Here's how the part is built. I have some questions about the finished solid (model axes, mm). Face numbers are marked on the shaded views. A direction names the side the tool comes from. Coordinates: 2 decimals unless noted, no trailing zeros. Loops run counter-clockwise (first coordinate to the right, second up) from the corner with the lowest first, then second, coordinate; pieces in that order, holes last. Notation, with made-up numbers: (3, 75) -> (54, 75) arc R23 cw to (54, 91) -> close; hole circle Ø6 at (36, 84). An arc over 180 degrees is marked (long way). Answer as a JSON object with one key per item and string values. Group by question number.
Q1. I want a section at B-B on y = 119.5. Write out the boundary of the cut face in (x, z).
Q2. I'm going to push flat-ended pins straight in: pin 1 (6 mm diameter, centred on x = 66, y = 139.5, fed in from -Z); pin 2 (8 mm diameter, centred on x = -52, y = -66, fed in from +Z). Where does each tip first touch, or does it pass through?
Q3. On a 3-axis mill with a long thin cutter (end or side, diameter ignored), from which of +Z, -Z, +X, -X, +Y, -Y can I reach the whole of each face in a straight line? I mean the marked faces 5 and 6. Say none if no direction works.
Q4. I want a section at A-A on z = 96. Write out the boundary of the cut face in (x, y), then the cut area to 3 significant figures.
Q5. I want a section at C-C on x = -93.5. Write out the boundary of the cut face in (y, z), then the cut area to 3 significant figures.
Q6. I need wall thicknesses on line 1 (X direction, y = 207, z = 84); line 2 (Y direction, x = 89.5, z = 202); line 3 (Y direction, x = -180.5, z = 237.5). Which ranges of each line are inside material? Lowest first, please.
Q7. Thinking about a two-plate mould opening in Y: for the marked faces 1, 2, 3 and 4, which applies, released by +Y, released by -Y, zero draft, split by the parting line, or undercut?
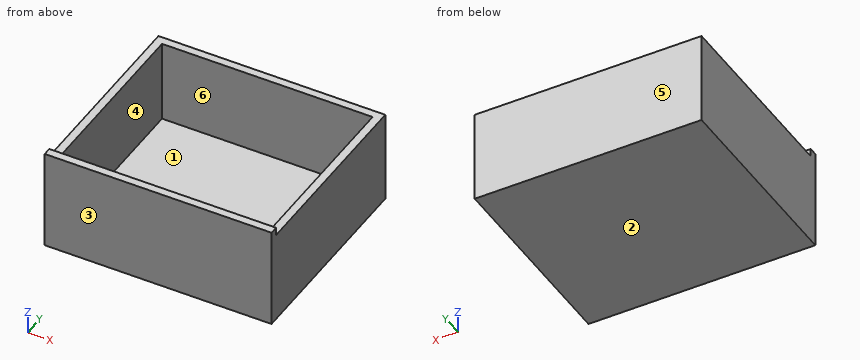
```python
from build123d import *

# Parameters (mm, degrees)
F0_W     = 20
F0_H     = 460
F0_H_2   = 20
F0_W_2   = 520
F1_DEPTH = 230
F2_DEPTH = 250
F3_DEPTH = 25


with BuildPart() as f1:
    # F0 (on Top) → F1 (new body)
    with BuildSketch(Plane.XY):
        with Locations((-270, 0)):
            Rectangle(F0_W, F0_H)
        with Locations((-270, 240)):
            Rectangle(F0_W, F0_H_2)
        with Locations((0, 240)):
            Rectangle(F0_W_2, F0_H_2)
        with Locations((270, 0)):
            Rectangle(F0_W, F0_H)
        with Locations((270, 240)):
            Rectangle(F0_W, F0_H_2)
    extrude(amount=F1_DEPTH)

    # F0 (on Top) → F2 (join)
    with BuildSketch(Plane.XY):
        with Locations((-270, -240)):
            Rectangle(F0_W, F0_H_2)
        with Locations((0, -240)):
            Rectangle(F0_W_2, F0_H_2)
        with Locations((270, -240)):
            Rectangle(F0_W, F0_H_2)
    extrude(amount=F2_DEPTH)

    # F0 (on Top) → F3 (join)
    with BuildSketch(Plane.XY):
        with Locations((270, -240)):
            Rectangle(F0_W, F0_H_2)
        with Locations((0, -240)):
            Rectangle(F0_W_2, F0_H_2)
        with Locations((270, 0)):
            Rectangle(F0_W, F0_H)
        with Locations((-270, -240)):
            Rectangle(F0_W, F0_H_2)
        with Locations((270, 240)):
            Rectangle(F0_W, F0_H_2)
        with Locations((-270, 0)):
            Rectangle(F0_W, F0_H)
        with Locations((0, 240)):
            Rectangle(F0_W_2, F0_H_2)
        with Locations((-270, 240)):
            Rectangle(F0_W, F0_H_2)
        Rectangle(F0_W_2, F0_H)
    extrude(amount=F3_DEPTH)


solid = f1.part
```
Result set:
{
 "1": {"outline": "(-280, 0) -> (280, 0) -> (280, 230) -> (260, 230) -> (260, 25) -> (-260, 25) -> (-260, 230) -> (-280, 230) -> close"},
 "2": {"pin 1": "stops at z = 0", "pin 2": "stops at z = 25"},
 "3": {"face 5": "+Z, -Z, +X, -X, +Y", "face 6": "+Z"},
 "4": {"outline": "(-280, -250) -> (280, -250) -> (280, 250) -> (-280, 250) -> close; hole (-260, -230) -> (260, -230) -> (260, 230) -> (-260, 230) -> close", "area": "40,800 mm²"},
 "5": {"outline": "(-250, 0) -> (250, 0) -> (250, 230) -> (230, 230) -> (230, 25) -> (-230, 25) -> (-230, 250) -> (-250, 250) -> close", "area": "21,100 mm²"},
 "6": {"line 1": "x = -280 to -260, 260 to 280", "line 2": "y = -250 to -230, 230 to 250", "line 3": "y = -250 to -230"},
 "7": {"face 1": "undercut", "face 2": "zero draft", "face 3": "released by -Y", "face 4": "undercut"}
}
